Input: part model. Units: mm. Frame: model coordinates. Face numbers are marked on the shaded views. A direction names the side the tool comes from. Give positions to 0.01 mm unless a question says otherwise; leave off trailing zeros. Loops run counter-clockwise (first coordinate to the right, second up) from the corner with the lowest first, then second, coordinate; pieces in that order, holes last.
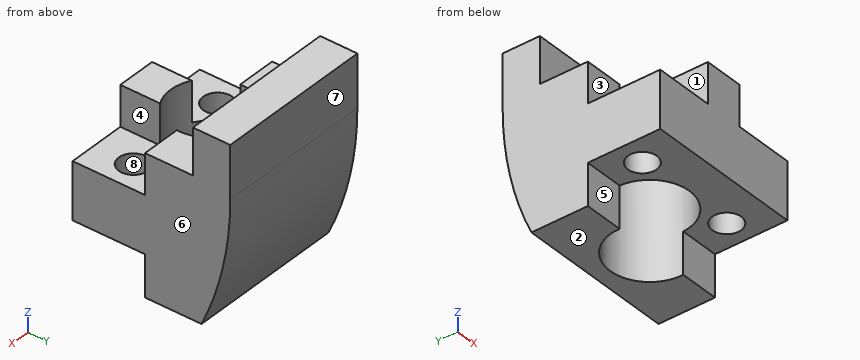
Solid Edge part; units mm, degrees
sketch "Sketch1" plane through (0, 0, 0) normal (0, -1, 0) x (1, 0, 0)
  line L0 (-19.05, -22.25) -> (19.05, -22.25)
  line L1 (19.05, -22.25) -> (19.05, 22.25)
  line L2 (19.05, 22.25) -> (-19.05, 22.25)
  line L3 (-19.05, 22.25) -> (-19.05, -22.25)
extrude "Protrusion1" add sketch "Sketch1" against normal blind 38.1
sketch "Sketch2" plane through (0, 0, 0) normal (0, -1, 0) x (1, 0, 0)
  line L0 (-19.05, 22.25) -> (-19.05, 11.15)
  line L1 (-19.05, 11.15) -> (19.05, 11.15)
  line L2 (19.05, 11.15) -> (19.05, 22.25)
  line L3 (19.05, 22.25) -> (-19.05, 22.25)
extrude "ExtrudedCutout_2" cut sketch "Sketch2" against normal blind 29.1
sketch "Sketch3" plane through (0, 0, -5.55) normal (0, -1, 0) x (1, 0, 0)
  line L0 (-19.05, 16.7) -> (-19.05, 7)
  line L1 (-19.05, 7) -> (-4.75, 7)
  line L2 (-4.75, 7) -> (-4.75, 16.7)
  line L3 (-4.75, 16.7) -> (-19.05, 16.7)
extrude "ExtrudedCutout_3" cut sketch "Sketch3" against normal blind 17.5
sketch "Sketch4" plane through (0, 0, -5.55) normal (0, -1, 0) x (1, 0, 0)
  line L0 (19.05, 16.7) -> (19.05, 7)
  line L1 (19.05, 7) -> (4.75, 7)
  line L2 (4.75, 7) -> (4.75, 16.7)
  line L3 (4.75, 16.7) -> (19.05, 16.7)
extrude "ExtrudedCutout_4" cut sketch "Sketch4" against normal blind 17.5
sketch "Sketch5" plane through (0, 0, 0) normal (0, -1, 0) x (1, 0, 0)
  line L0 (-19.05, -22.25) -> (-19.05, -12.25)
  line L1 (-19.05, -12.25) -> (19.05, -12.25)
  line L2 (19.05, -12.25) -> (19.05, -22.25)
  line L3 (19.05, -22.25) -> (-19.05, -22.25)
extrude "ExtrudedCutout_8" cut sketch "Sketch5" against normal blind 17.5
sketch "Sketch6" plane through (0, 0, 0) normal (0, 0, 1) x (1, 0, 0)
  circle A0 centre (-12.65, 9.5) radius 3.5
  circle A1 centre (12.65, 9.5) radius 3.5
extrude "Cutout1" cut sketch "Sketch6" against normal up to vertex (12.25 mm away)
sketch "Sketch7" plane through (0, 0, 0) normal (0, 0, 1) x (1, 0, 0)
  circle A0 centre (-12.65, 9.5) radius 3.5
extrude "Cutout2" cut sketch "Sketch7" along normal blind 20
sketch "Sketch8" plane through (0, 0, 0) normal (0, 0, 1) x (1, 0, 0)
  circle A0 centre (12.65, 9.5) radius 3.5
extrude "ExtrudedCutout_16" cut sketch "Sketch8" along normal blind 20
sketch "Sketch9" plane through (19.05, 19.05, 0) normal (1, 0, 0) x (0, 1, 0)
  arc A0 (19.05, 9.55) -> (12.0974, -22.25) centre (-57.15, 9.55) cw
  line L0 (12.0974, -22.25) -> (19.05, -22.25)
  line L1 (19.05, -22.25) -> (19.05, 9.55)
extrude "ExtrudedCutout_17" cut sketch "Sketch9" against normal blind 40
sketch "Sketch10" plane through (0, 14.55, 11.15) normal (0, 0, 1) x (1, 0, 0)
  circle A0 centre (0, 3.35) radius 9.55
extrude "Cutout3" cut sketch "Sketch10" against normal blind 98
(1) Ray query, probe 1 along X at (y, z) = (17.9, 3.5); probe 2 along X at (y, z) = (9.5, -6); probe 3 along Y at (x, z) = (0, 9). Return the intervals inside material, ascending.
Values follow:
probe 1: x = -19.05 to -9.55, 9.55 to 19.05
probe 2: x = -19.05 to -16.15, -9.15 to -4.54, 4.54 to 9.15, 16.15 to 19.05
probe 3: y = 0 to 8.35, 27.45 to 38.1
(2) Cut plane D-D (z = -9). Return the cut outline in (x, y).
Values follow:
outline: (-19.05, 0) - (19.05, 0) - (19.05, 35.81) - (-19.05, 35.81) - close; hole circle Ø7 at (-12.65, 9.5); hole circle Ø19.1 at (0, 17.9); hole circle Ø7 at (12.65, 9.5)
(3) Cut plane B-B (z = 10.5). Return the cut outline in (x, y).
Values follow:
outline: (-19.05, 17.5) - (-9.54, 17.5) arc R9.55 cw (long way) to (9.54, 17.5) - (19.05, 17.5) - (19.05, 38.1) - (-19.05, 38.1) - close; (-4.75, 0) - (4.75, 0) - (4.75, 9.62) arc R9.55 cw to (-4.75, 9.62) - close
(4) Cut plane C-C (y = 20). Return the cut outline in (x, z), and give its area (3 significant figures).
Values follow:
outline: (-19.05, -22.25) - (-9.32, -22.25) - (-9.32, 11.15) - (-19.05, 11.15) - close; (9.32, -22.25) - (19.05, -22.25) - (19.05, 11.15) - (9.32, 11.15) - close
area: 650 mm2
(5) Reachability of the marked faces 1, 2, 3, 4 and 5 from +Z, -Z, +X, -X, +Y, -Y: full face, straight path, thin tool, end or side. Return the list, or none.
Values follow:
face 1: +Z, -X, -Y
face 2: -Z, +X, -X, +Y, -Y
face 3: +Z, +X, -X, -Y
face 4: +Z, +X, -Y
face 5: -Z, +X, -X, -Y
(6) Pin query (flat end, axial travel): pin 1 Ø15.5 at (x, y) = (9, 8.5) entering from +Z; pin 2 Ø8 at (x, y) = (-12.65, 9.5) entering from -Z; pin 3 Ø6 at (x, z) = (10.5, 12.5) entering from -Y. Return the tip coordinate at first contact, or that it passes through.
Values follow:
pin 1: stops at z = 11.15
pin 2: stops at z = -12.25
pin 3: stops at y = 17.5
(7) Cut plane A-A (x = 0). Return the cut outline in (y, z).
Values follow:
outline: (0, -12.25) - (8.35, -12.25) - (8.35, 11.15) - (0, 11.15) - close; (27.45, -22.25) - (31.15, -22.25) arc R76.2 ccw to (38.1, 9.55) - (38.1, 22.25) - (29.1, 22.25) - (29.1, 11.15) - (27.45, 11.15) - close
(8) Mould query, pull axis Y, two halves, no side actions, for the marked faces 6, 7 and 8. Classes: +Y half, -Y half, draft (parallel to the pull), parting line (faces both ways), or undercut.
Values follow:
face 6: draft
face 7: +Y half
face 8: undercut
